Read the model definition and answer for the solid it produces. Units are mm, in the model's axes. A direction names the side the tool comes from. Coordinates: 2 decimals unless noted, no trailing zeros. Loops run counter-clockwise (first coordinate to the right, second up) from the corner with the lowest first, then second, coordinate; pieces in that order, holes last.
Q1. The mould has two halves that part along Y. Classify faces 5 (the face through (232, -156.913, 4)), 6 (the face through (223.659, -151, 4)), 7 (the face through (88, -106.913, 4)): pulls with the +Y half, pulls with the -Y half, needs draft (parallel to the pull), parting line crosses it, or undercut.
Q2. Section B-B (x = 169.5) is taken. Give the vertices of the cut face in (y, z).
Q3. Straight lines are drawn through the part: line 1 (Y direction, x = 98, z = 2.25); line 2 (X direction, y = -8, z = 0.75); line 3 (Y direction, x = -37.5, z = 4). For each, find the intervals that lie inside material, in ascending order.
Q4. Which of the six approach directions +Z, -Z, +X, -X, +Y, -Y give full straight-line access (tool end or side, diameter ignored) to faces 1 (the face through (-52, -156.913, 4)), 2 (the face through (-43.841, -151, 4)), 3 (the face through (224.159, 137, 4)), 4 (the face through (88, 132, 4))?
Q5. Section A-A (y = 79) is taken. Give the vertices of the cut face in (x, z), then the cut area to 3 significant figures.
Q6. A flat-ended cylindrical pin translates along its axis: P1, Ø3, axis at y = -152.91, z = 4, coming from the -X side. Find the tip coordinate at first contact, or state that the pin passes through.
from build123d import *
from build123d.topology import SkipClean

# Parameters (mm, degrees)
SKETCH1_R                       = 1.5
SKETCH1_W                       = 200
SKETCH1_H                       = 4
BOSS_EXTRUDE1_DEPTH             = 8
M4_TAPPED_HOLE1_D               = 3.3
M4_TAPPED_HOLE1_DEPTH           = 25
M4_TAPPED_HOLE1_TIP             = 0.991420021
M4_TAPPED_HOLE1_ON_FACE_2_D     = 3.3
M4_TAPPED_HOLE1_ON_FACE_2_DEPTH = 25
M4_TAPPED_HOLE1_ON_FACE_2_TIP   = 0.991420021


with BuildPart() as part:
    # Sketch1 → Boss-Extrude1 (new body)
    with BuildSketch(Plane.XY):
        with BuildLine():
            Line((179.658803725, 93.087327907), (179.658803725, -6.912672093))
            Line((179.658803725, -6.912672093), (206.158803725, -6.912672093))
            ThreePointArc((206.158803725, -6.912672093), (217.658803725, 4.587327907), (229.158803725, -6.912672093))
            Line((229.158803725, -6.912672093), (239.658803725, -6.912672093))
            Line((239.658803725, -6.912672093), (239.658803725, 143.087327907))
            Line((239.658803725, 143.087327907), (224.158803725, 143.087327907))
            Line((224.158803725, 143.087327907), (224.158803725, 133.066458278))
            ThreePointArc((224.158803725, 133.066458278), (223.408586049, 121.092547584), (223.658803725, 133.087327907))
            Line((223.658803725, 133.087327907), (223.658803725, 143.087327907))
            Line((223.658803725, 143.087327907), (-43.841196275, 143.087327907))
            Line((-43.841196275, 143.087327907), (-43.841196275, 133.066458278))
            ThreePointArc((-43.841196275, 133.066458278), (-44.341196275, 121.087327907), (-44.841196275, 133.066458278))
            Line((-44.841196275, 133.066458278), (-44.841196275, 143.087327907))
            Line((-44.841196275, 143.087327907), (-60.341196275, 143.087327907))
            Line((-60.341196275, 143.087327907), (-60.341196275, -6.912672093))
            Line((-60.341196275, -6.912672093), (-49.841196275, -6.912672093))
            ThreePointArc((-49.841196275, -6.912672093), (-38.341196275, 4.587327907), (-26.841196275, -6.912672093))
            Line((-26.841196275, -6.912672093), (-0.341196275, -6.912672093))
            Line((-0.341196275, -6.912672093), (-0.341196275, 93.087327907))
            Line((-0.341196275, 93.087327907), (179.658803725, 93.087327907))
        make_face()
        with Locations((-53.841196275, 8.587327907)):
            Circle(SKETCH1_R, mode=Mode.SUBTRACT)
        with Locations((-22.841196275, 8.587327907)):
            Circle(SKETCH1_R, mode=Mode.SUBTRACT)
        with Locations((233.158803725, 8.587327907)):
            Circle(SKETCH1_R, mode=Mode.SUBTRACT)
        with Locations((202.158803725, 8.587327907)):
            Circle(SKETCH1_R, mode=Mode.SUBTRACT)
        with Locations((89.658803725, 134)):
            Rectangle(SKETCH1_W, SKETCH1_H, mode=Mode.SUBTRACT)
    boss_extrude1 = extrude(amount=BOSS_EXTRUDE1_DEPTH)

    # Mirror1: Boss-Extrude1 across plane
    with SkipClean():  # the faces are left unmerged after this step: merging them gives an invalid solid
        add(boss_extrude1.mirror(Plane(origin=(0, -6.912672093, 8), x_dir=(0, 0, 1), z_dir=(0, 1, 0))))

    # M4 Tapped Hole1
    with Locations(Plane(origin=(-60.341196275, -152.912672093, 4), x_dir=(0, 0, -1), z_dir=(-1, 0, 0))):
        with Locations((0, 0), (0, -292)):
            Hole(M4_TAPPED_HOLE1_D / 2, depth=M4_TAPPED_HOLE1_DEPTH)
            with Locations((0, 0, -(M4_TAPPED_HOLE1_DEPTH + M4_TAPPED_HOLE1_TIP / 2))):  # 118° drill point
                Cone(0, M4_TAPPED_HOLE1_D / 2, M4_TAPPED_HOLE1_TIP, mode=Mode.SUBTRACT)

    # M4 Tapped Hole1 on face 2
    with Locations(Plane(origin=(239.658803725, -152.912672093, 4), x_dir=(0, 0, 1), z_dir=(1, 0, 0))):
        with Locations((0, 0), (0, -292)):
            Hole(M4_TAPPED_HOLE1_ON_FACE_2_D / 2, depth=M4_TAPPED_HOLE1_ON_FACE_2_DEPTH)
            with Locations((0, 0, -(M4_TAPPED_HOLE1_ON_FACE_2_DEPTH + M4_TAPPED_HOLE1_ON_FACE_2_TIP / 2))):  # 118° drill point
                Cone(0, M4_TAPPED_HOLE1_ON_FACE_2_D / 2, M4_TAPPED_HOLE1_ON_FACE_2_TIP, mode=Mode.SUBTRACT)


solid = part.part
Numbers:
1. face 5: pulls with the -Y half
1. face 6: needs draft
1. face 7: undercut
2. outline: (-156.91, 0) - (-149.83, 0) - (-149.83, 8) - (-156.91, 8) - close; (-145.83, 0) - (-106.91, 0) - (-106.91, 8) - (-145.83, 8) - close; (93.09, 0) - (132, 0) - (132, 8) - (93.09, 8) - close; (136, 0) - (143.09, 0) - (143.09, 8) - (136, 8) - close
3. line 1: y = -156.91 to -149.83, -145.83 to -106.91, 93.09 to 132, 136 to 143.09
3. line 2: x = -60.34 to -49.79, -26.89 to -0.34, 179.66 to 206.21, 229.11 to 239.66
3. line 3: y = -156.91 to -154.56, -151.26 to -18.38, 4.56 to 137.44, 140.74 to 143.09
4. face 1: +Z, -Z, +X, -X, -Y
4. face 2: +Z, -Z, -Y
4. face 3: +Z, -Z, +Y
4. face 4: +Z, -Z
5. outline: (-60.34, 0) - (-0.34, 0) - (-0.34, 8) - (-60.34, 8) - close; (179.66, 0) - (239.66, 0) - (239.66, 8) - (179.66, 8) - close
5. area: 960 mm2
6. P1: stops at x = -35.25
